Solid Edge part; units mm, degrees
sketch "Sketch1" plane through (0, 0, 0) normal (0, -1, 0) x (1, 0, 0)
  line L0 (22.5, 36.5) -> (22.5, -33)
  line L1 (22.5, -33) -> (-22.5, -33)
  line L2 (-22.5, -33) -> (-22.5, 36.5)
  line L3 (-22.5, 36.5) -> (22.5, 36.5)
  circle A0 centre (0, 28) radius 6
  circle A1 centre (0, 8) radius 4.6
extrude "Protrusion1" add sketch "Sketch1" against normal blind 10
sketch "Sketch2" plane through (0, 10, 4.6) normal (0, 1, 0) x (-1, 0, 0)
  circle A0 centre (0, 3.4) radius 11.25
extrude "ExtrudedCutout_1" cut sketch "Sketch2" against normal blind 7.5
sketch "Sketch3" plane through (0, 5, -33) normal (0, 0, -1) x (1, 0, 0)
  circle A0 centre (-17.5, 0) radius 2.5
extrude "ExtrudedCutout_2" cut sketch "Sketch3" against normal blind 10
sketch "Sketch4" plane through (0, 2.5, 8) normal (0, 1, 0) x (-1, 0, 0)
  circle A0 centre (0, 0) radius 4.6
extrude "Protrusion2" add sketch "Sketch4" against normal up to vertex (2.5 mm away)
sketch "Sketch5" plane through (0, 5, -33) normal (0, 0, -1) x (1, 0, 0)
  circle A0 centre (17.5, 0) radius 2.5
extrude "ExtrudedCutout_3" cut sketch "Sketch5" against normal blind 10
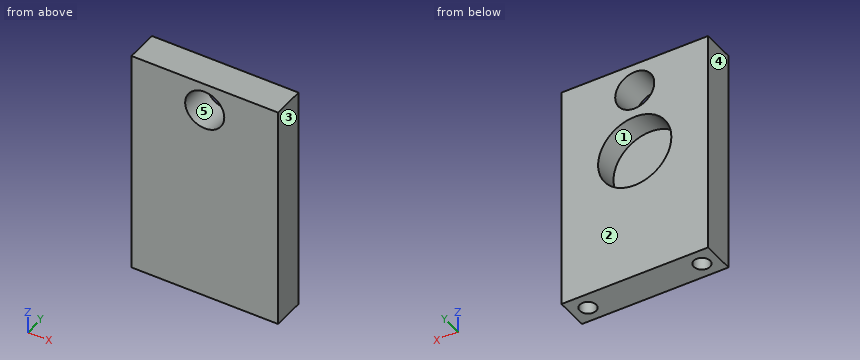
Model file for the job. Use its own axes, mm. Face numbers are marked on the shaded views. A direction names the side the tool comes from. Coordinates: 2 decimals unless noted, no trailing zeros. Loops run counter-clockwise (first coordinate to the right, second up) from the corner with the lowest first, then second, coordinate; pieces in that order, holes last. Notation, with made-up numbers: (49.25, 30) -> (102.25, 30) arc R28 ccw to (102.25, 53) -> close; hole circle Ø10 at (-30, -20.5). An arc over 180 degrees is marked (long way). Use one line per item in the form item = value. Start each with the question number.
(1) Probe probe 1 along Z at (x, y) = (0, 5); probe 2 along X at (y, z) = (5, -28.75); probe 3 along X at (y, z) = (7.25, 7.5). List the from-to ranges inside material, lowest first. Write a range as from..to.
(2) Cut at D-D on z = 8. Give the cut face in (x, y), and give its area (3 significant figures).
(3) Cut at C-C on x = -16. Give the cut face in (y, z).
(4) Flat gauge pins, fed straight in: pin 1 (7 mm diameter, centred on x = -5.5, z = 4.5, fed in from +Y); pin 2 (2.5 mm diameter, centred on x = -18, y = 6, fed in from -Z). Where does each tip first touch, or does it go through?
(5) Cut at B-B on y = 1.5. Give the cut face in (x, z), and give its area (3 significant figures).
(6) Cut at A-A on x = 0. Give the cut face in (y, z).
(7) Pull direction X, two halves, no side cores. Call the marked faces 3, 4 and 5: pulls with the +X half, pulls with the -X half, needs draft (parallel to the pull), parting line crosses it, or undercut.
(8) Tool access for the marked faces 1 and 2: list every direction of +Z, -Z, +X, -X, +Y, -Y with a clear straight run to the whole face (end or side of a thin tool).
Values:
q1.probe_1 = -33..-3.25, 19.25..22, 34..36.5
q1.probe_2 = -22.5..-20, -15..15, 20..22.5
q1.probe_3 = -22.5..-11.24, 11.24..22.5
q2.outline = (-22.5, 0) -> (22.5, 0) -> (22.5, 10) -> (11.25, 10) -> (11.25, 2.5) -> (-11.25, 2.5) -> (-11.25, 10) -> (-22.5, 10) -> close
q2.area = 281 mm2
q3.outline = (0, -33) -> (3, -33) -> (3, -23) -> (7, -23) -> (7, -33) -> (10, -33) -> (10, 36.5) -> (0, 36.5) -> close
q4.pin_1 = 2.5
q4.pin_2 = -23
q5.outline = (-22.5, -33) -> (22.5, -33) -> (22.5, 36.5) -> (-22.5, 36.5) -> close; hole circle Ø12 at (0, 28)
q5.area = 3,010 mm2
q6.outline = (0, -33) -> (10, -33) -> (10, -3.25) -> (2.5, -3.25) -> (2.5, 19.25) -> (10, 19.25) -> (10, 22) -> (0, 22) -> close; (0, 34) -> (10, 34) -> (10, 36.5) -> (0, 36.5) -> close
q7.face_3 = pulls with the +X half
q7.face_4 = pulls with the -X half
q7.face_5 = undercut
q8.face_1 = +Y
q8.face_2 = +Z, -Z, +X, -X, +Y
